Verification items for this drawing (mm, ordinates from the low corner). A direction names the side the tool comes from. Give positions to 0.01 mm unless a question says otherwise; leave off trailing zeros. Order: outer loops, then holes, each group sorted by start corner. A loop starts at its lowest first (then second) coordinate and runs counter-clockwise, first axis right, second up.
(1) Access from +Z, -Z, +X, -X, +Y, -Y to the whole of each face (thin tool, end or side, straight path). Record for the marked faces 1 and 2.
(2) Sectioned sample at C-C on z = 8.75. Record the cut outline in (x, y), plus the area to 3 significant figures.
(3) Sectioned sample at A-A on x = 12. Record the cut outline in (y, z).
(4) Scan lines: L1, parallel to Y at x = 12, z = 13.95; L2, parallel to X at y = 74.5, z = 2.75; L3, parallel to Z at x = 14.5, y = 25. Record each from-to range of solid material in increasing order.
(5) Sectioned sample at D-D on y = 50. Record the cut outline in (x, z), plus the area to 3 significant figures.
(6) Sectioned sample at B-B on y = 10. Record the cut outline in (x, z), plus the area to 3 significant figures.
(7) Gauge pin test, flat ends, axial feed: pin 1 (5 mm diameter, centred on x = 12, y = 30, fed in from +Z); pin 2 (2.5 mm diameter, centred on x = 12, y = 10, fed in from +Z); pin 3 (6.5 mm diameter, centred on x = 12, y = 90, fed in from -Z). Record the tip position at first contact, or that the pin passes through.
(8) Mould release check, pull along X, two halves, no side actions. Record for the marked faces 3, 4, 5 and 6: pulls with the +X half, pulls with the -X half, needs draft (parallel to the pull), parting line crosses it, or undercut.
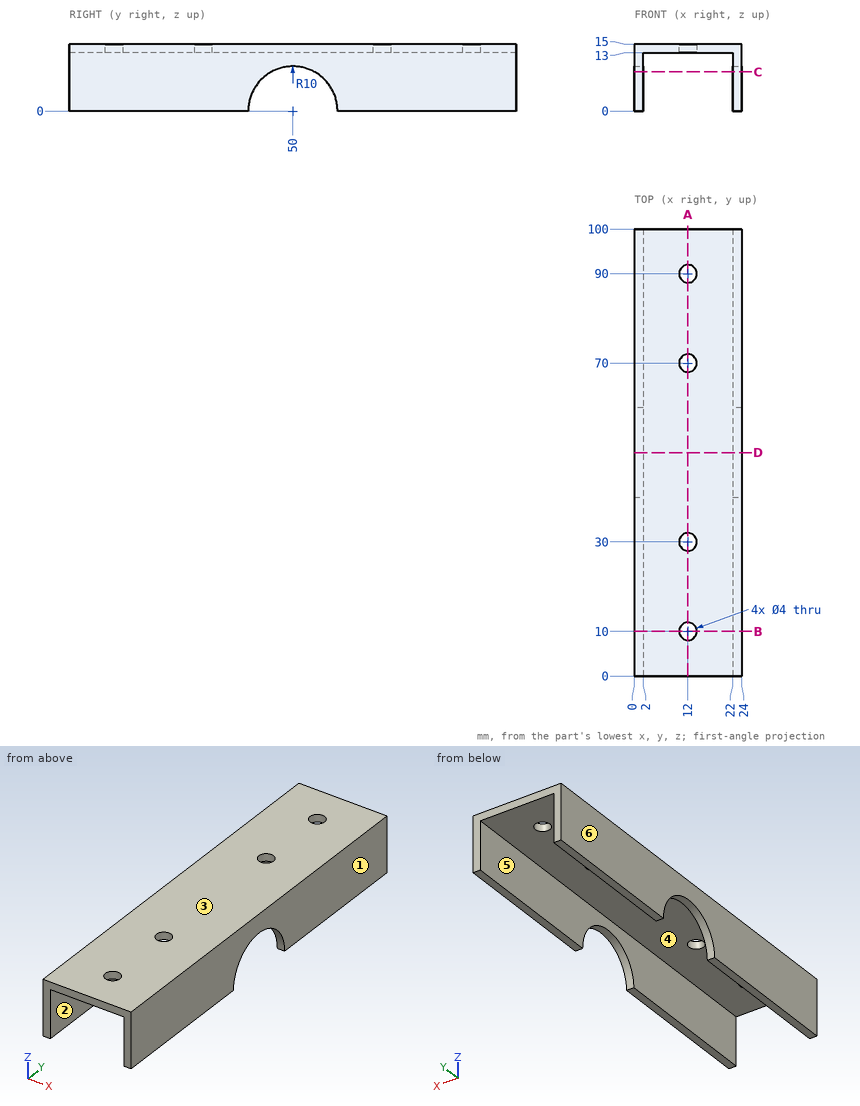
Ans:
1. face 1: +Z, -Z, +X, +Y, -Y
1. face 2: -Z, +Y, -Y
2. outline: (0, 0) - (2, 0) - (2, 45.16) - (0, 45.16) - close; (0, 54.84) - (2, 54.84) - (2, 100) - (0, 100) - close; (22, 0) - (24, 0) - (24, 45.16) - (22, 45.16) - close; (22, 54.84) - (24, 54.84) - (24, 100) - (22, 100) - close
2. area: 361 mm2
3. outline: (0, 13) - (8, 13) - (8, 15) - (0, 15) - close; (12, 13) - (28, 13) - (28, 15) - (12, 15) - close; (32, 13) - (68, 13) - (68, 15) - (32, 15) - close; (72, 13) - (88, 13) - (88, 15) - (72, 15) - close; (92, 13) - (100, 13) - (100, 15) - (92, 15) - close
4. L1: y = 0 to 8, 12 to 28, 32 to 68, 72 to 88, 92 to 100
4. L2: x = 0 to 2, 22 to 24
4. L3: z = 13 to 15
5. outline: (0, 10) - (2, 10) - (2, 13) - (22, 13) - (22, 10) - (24, 10) - (24, 15) - (0, 15) - close
5. area: 60.0 mm2
6. outline: (0, 0) - (2, 0) - (2, 13) - (10, 13) - (10, 15) - (0, 15) - close; (14, 13) - (22, 13) - (22, 0) - (24, 0) - (24, 15) - (14, 15) - close
6. area: 92.0 mm2
7. pin 1: stops at z = 15
7. pin 2: passes through
7. pin 3: stops at z = 13
8. face 3: needs draft
8. face 4: undercut
8. face 5: undercut
8. face 6: pulls with the -X half
